Read the model definition and answer for the solid it produces. Units are mm, in the model's axes. Face numbers are marked on the shaded views. Coordinates: 2 decimals unless noted, no trailing zeros. Loops run counter-clockwise (first coordinate to the right, second up) from the corner with the lowest first, then second, coordinate; pieces in that order, holes last.
Autodesk Inventor part; units mm, degrees
ref_plane "YZ Plane" through (0, 0, 0) normal (1, 0, 0) x (0, 1, 0)
ref_plane "XZ Plane" through (0, 0, 0) normal (0, 1, 0) x (-1, 0, 0)
ref_plane "XY Plane" through (0, 0, 0) normal (0, 0, 1) x (1, 0, 0)
sketch "Sketch1" plane through (0, 0, 0) normal (0, 1, 0) x (-1, 0, 0)
  arc A0 (6, 0) -> (-6, 0) centre (0, 0) ccw
  line L0 (6, 0) -> (6, -12.3)
  line L1 (4.2426, -16.5426) -> (-8.4574, -29.2426)
  line L2 (-16.9426, -20.7574) -> (-6, -9.8147)
  line L3 (-6, -9.8147) -> (-6, 0)
  arc A1 (-16.9426, -20.7574) -> (-8.4574, -29.2426) centre (-12.7, -25) ccw
  arc A2 (4.2426, -16.5426) -> (6, -12.3) centre (0, -12.3) ccw
  line L4 (0, 0) -> (-12.7, -25) construction
  circle A3 centre (0, 0) radius 6
  circle A4 centre (-12.7, -25) radius 6
  arc A5 (-10.3351, -19.4857) -> (-3.0586, -5.1619) centre (-7.1622, -12.0874) ccw
  arc A6 (-15.0649, -30.5143) -> (3.0586, 5.1619) centre (-7.1622, -12.0874) ccw
  point P0 (6, -14.7853)
  point P1 (-16.9426, -20.7574)
  point P2 (-15.0649, -30.5143)
  point P3 (3.0586, 5.1619)
  point P4 (-6, 0)
  dimension "d0" = 12
  dimension "d1" = 12.7
  dimension "d2" = 25
  dimension "d3" = 135
  dimension "d6" = 6
  dimension "d17" = 8.05
extrude "Extrusion1" add sketch "Sketch1" along normal blind 6 contours A3 A0 | A0 A6 A1 L1 A2 L0 | L0 A2 L1 A4 A5 A3 | A1 A4
sketch "Sketch2" plane through (0, 6, 0) normal (0, 1, 0) x (1, 0, 0)
  arc A0 (10.3351, 19.4857) -> (15.0649, 30.5143) centre (12.7, 25) ccw
  point P0 (0, 0)
  point P1 (16.9426, 20.7574)
  point P2 (8.4574, 29.2426)
hole "Hole1" at (0, 6, 0) at (12.7, 6, -25) direction (0, -1, 0) diameter 6.7564 depth 12.7 tip angle 118
properties part number "Tensioner2"
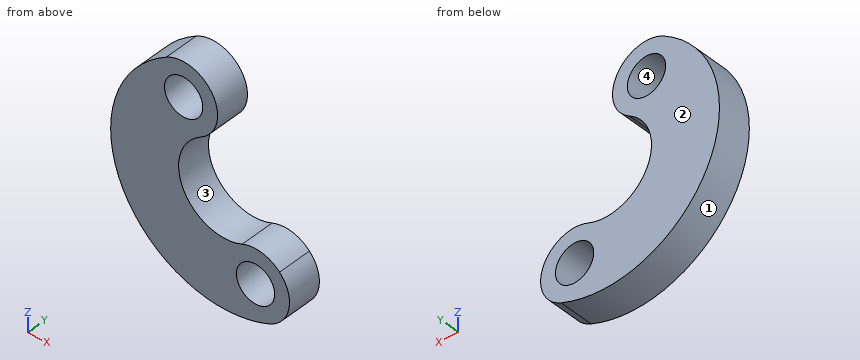
Item 1: Determine the mould class of the marked faces 1, 2, 3 and 4 for opening direction Z: released by +Z, released by -Z, zero draft, split by the parting line, or undercut.
Numbers:
face 1: split by the parting line
face 2: zero draft
face 3: undercut
face 4: undercut
Item 2: Find the intervals of material crossed by line 1 along Z through (x, y) = (0, 3.7); line 2 along Z through (x, y) = (-3, 4.55); line 3 along Z through (x, y) = (12.7, 2.3), in increasing order.
Numbers:
line 1: z = -30.81 to -15.76, -8.41 to -3.38, 3.38 to 6
line 2: z = -29.37 to -1.55, 1.55 to 5.2
line 3: z = -31.36 to -28.38, -21.62 to -19
Item 3: A cutting plane is placed at A-A on z = -1.5. Determine the outline of the cut face in (x, y).
Numbers:
outline: (-9.86, 0) - (-3.03, 0) - (-3.03, 6) - (-9.86, 6) - close; (3.03, 0) - (5.81, 0) - (5.81, 6) - (3.03, 6) - close
Item 4: A cutting plane is placed at C-C on x = 0. Determine the outline of the cut face in (y, z).
Numbers:
outline: (0, -30.81) - (6, -30.81) - (6, -15.76) - (0, -15.76) - close; (0, -8.41) - (6, -8.41) - (6, -3.38) - (0, -3.38) - close; (0, 3.38) - (6, 3.38) - (6, 6) - (0, 6) - close
Item 5: A cutting plane is placed at B-B on x = 12.7. Determine the outline of the cut face in (y, z).
Numbers:
outline: (0, -31.36) - (6, -31.36) - (6, -28.38) - (0, -28.38) - close; (0, -21.62) - (6, -21.62) - (6, -19) - (0, -19) - close
Item 6: Given pin 1 (2 mm diameter, centred on y = 5.5, z = -7.5, fed in from +X), flat-ended and moving along its own axis, determine where the tip first touches the part or whether it passes through.
Numbers:
pin 1: stops at x = 1.37
